CAD build for the part. Positions are in the model's coordinates, mm. Round coordinates to 2 decimals unless told otherwise and drop trailing zeros. Order: outer loops, then holes, each group sorted by start corner. A loop starts at its lowest first (then second) coordinate and runs counter-clockwise, first axis right, second up. Notation, with made-up numbers: (63, 40) -> (95, 40) arc R30 ccw to (95, 68) -> close; hole circle Ø3 at (11, -6.75). An arc over 180 degrees is marked (long way). Return JSON: item names as keys, results as strings. Group by question number.
Q1. Cut at A-A (z = 5). Write the cut outline in (x, y), then the cut area to 3 significant figures.
Q2. Cut at B-B (y = -18.5). Write the cut outline in (x, z), then the cut area to 3 significant figures.
Q3. Probe line 1 along X through (y, z) = (-7.5, 2.25). List the from-to ranges inside material, lowest first.
Q4. Flat gauge pins, fed straight in: pin 1 (2 mm diameter, centred on y = -4, z = 1, fed in from +X); pin 2 (1 mm diameter, centred on x = -3, z = 2.5, fed in from +Y); pin 3 (3 mm diameter, centred on x = 2.5, y = -7.5, fed in from -Z). Where does each tip first touch, or does it go through?
from build123d import *

# Parameters (mm, degrees)
F0_W     = 6.35
F0_H     = 38.1
F1_DEPTH = 6.35
F2_R     = 0.127
F3_DEPTH = 12.7
F4_DEPTH = 6.35


with BuildPart() as f1:
    # F0 (on Top) → F1 (new body)
    with BuildSketch(Plane.XY):
        with Locations((-11.249706, -2.776845)):
            Rectangle(F0_W, F0_H)
    extrude(amount=F1_DEPTH)

    # F2 (on face) → F3 (join)
    with BuildSketch(Plane.YZ.offset(-8.074706)):
        with Locations((-3.175, 2.026659)):
            Circle(F2_R)
        with Locations((-6.35, 2.026659)):
            Circle(F2_R)
        with Locations((-9.525, 2.026659)):
            Circle(F2_R)
        with Locations((-12.7, 2.026659)):
            Circle(F2_R)
        with Locations((-15.875, 2.026659)):
            Circle(F2_R)
    extrude(amount=F3_DEPTH)

    # F2 (on face) → F4 (join)
    with BuildSketch(Plane.YZ.offset(-8.074706)):
        with Locations((12.7, 2.026659)):
            Circle(F2_R)
        with Locations((9.525, 2.026659)):
            Circle(F2_R)
        with Locations((6.35, 2.026659)):
            Circle(F2_R)
        with Locations((3.175, 2.026659)):
            Circle(F2_R)
        with Locations((0, 2.026659)):
            Circle(F2_R)
    extrude(amount=F4_DEPTH)


solid = f1.part
Solution:
{
 "1": {"outline": "(-14.42, -21.83) -> (-8.07, -21.83) -> (-8.07, 16.27) -> (-14.42, 16.27) -> close", "area": "242 mm²"},
 "2": {"outline": "(-14.42, 0) -> (-8.07, 0) -> (-8.07, 6.35) -> (-14.42, 6.35) -> close", "area": "40.3 mm²"},
 "3": {"line 1": "x = -14.42 to -8.07"},
 "4": {"pin 1": "stops at x = -8.07", "pin 2": "stops at y = 12.83", "pin 3": "stops at z = 1.9"}
}
